Input: dimensioned drawing with shaded views. Units: mm. Origin: part minimum x, y, z. Give positions to 0.01 mm unless a question says otherwise; leave off trailing zeros. Write each loop counter-clockwise with the first axis right and the second up, starting at its lowest first coordinate (ties: lowest second). Pieces come first, ordered by that corner, then holes. Notation, with made-up numbers: (-35, 48.5) - (4, 48.5) arc R13 cw to (4, 54.5) - close; hole circle Ø10 at (15, -20.75). An arc over 180 degrees is marked (long way). Answer as CSV lines item,"result".
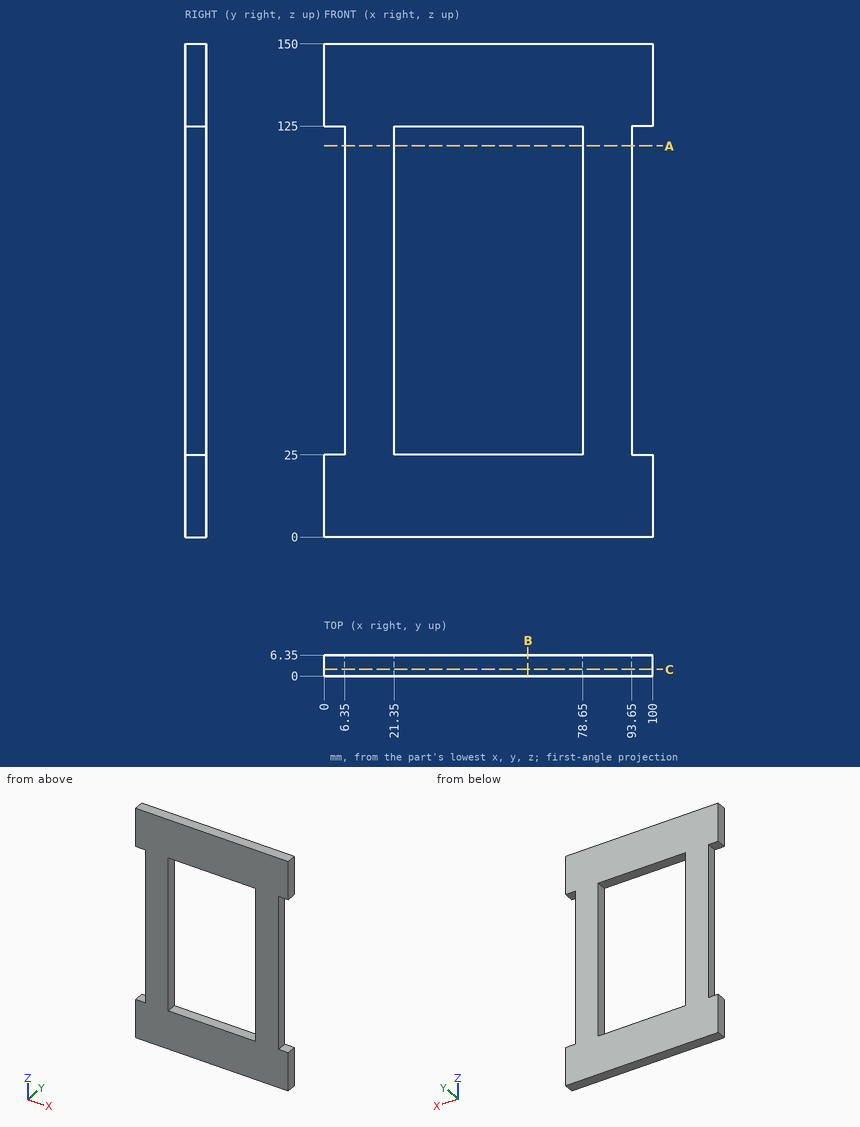
Item 1: Contact query for a flat-ended pin moving along its axis: pin 1 (3 mm diameter, centred on y = 4.5, z = 88.5, fed in from -X). Output: stop coordinate, or through.
The answers:
pin 1,"x = 6.35"
Item 2: Ray query, line 1 (Z direction, x = 21.5, y = 2); line 2 (X direction, y = 2, z = 85.5). Return the intervals inside material, ascending. Write a range as from..to.
The answers:
line 1,"0..25, 125..150"
line 2,"6.35..21.35, 78.65..93.65"
Item 3: Cut plane C-C on y = 2. Return the cut outline in (x, z), plus the area to 3 significant figures.
The answers:
outline,"(0, 0) - (100, 0) - (100, 25) - (93.65, 25) - (93.65, 125) - (100, 125) - (100, 150) - (0, 150) - (0, 125) - (6.35, 125) - (6.35, 25) - (0, 25) - close; hole (21.35, 25) - (78.65, 25) - (78.65, 125) - (21.35, 125) - close"
area,"8,000 mm²"
Item 4: Cut plane B-B on x = 62. Return the cut outline in (y, z), plus the area to 4 significant figures.
The answers:
outline,"(0, 0) - (6.35, 0) - (6.35, 25) - (0, 25) - close; (0, 125) - (6.35, 125) - (6.35, 150) - (0, 150) - close"
area,"317.5 mm²"
Item 5: Cut plane A-A on z = 119. Return the cut outline in (x, y), plus the area to 4 significant figures.
The answers:
outline,"(6.35, 0) - (21.35, 0) - (21.35, 6.35) - (6.35, 6.35) - close; (78.65, 0) - (93.65, 0) - (93.65, 6.35) - (78.65, 6.35) - close"
area,"190.5 mm²"
